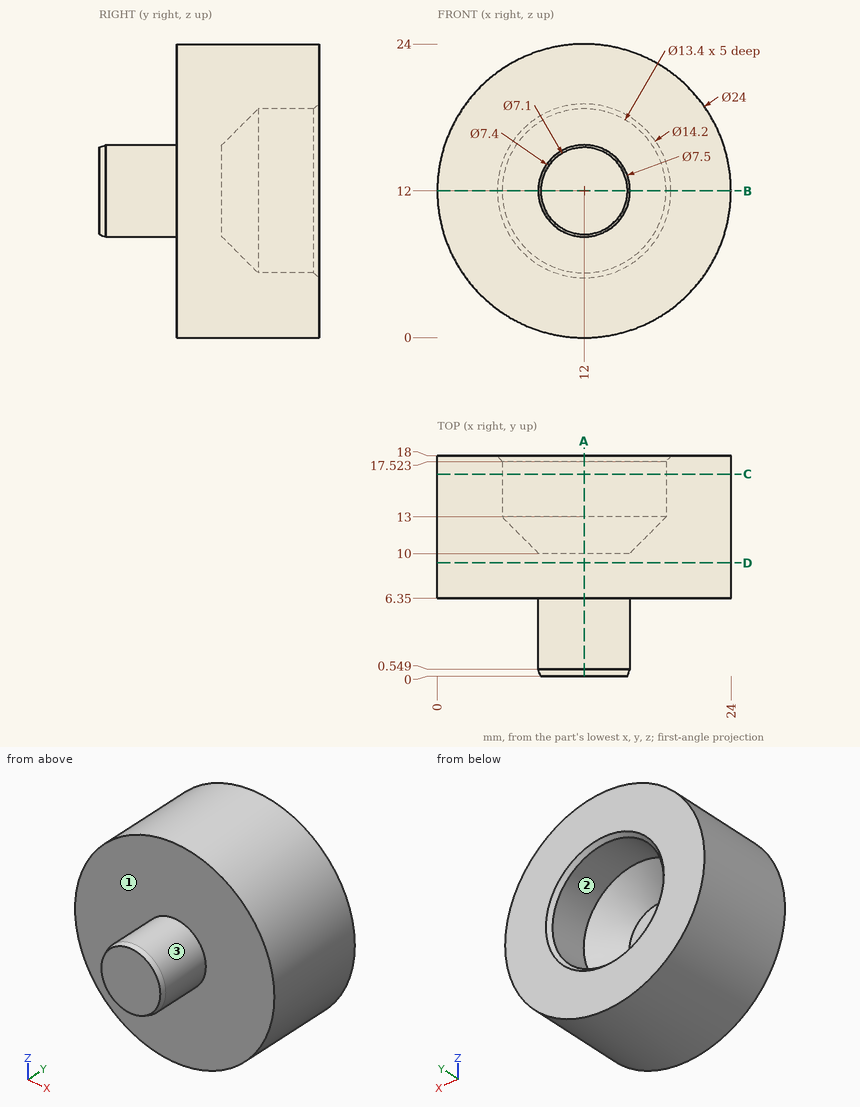
Job drawing, mm, ordinate dimensions from the low corner. One solid piece. Coordinates: 2 decimals unless noted, no trailing zeros. Order: outer loops, then holes, each group sorted by start corner. A loop starts at its lowest first (then second) coordinate and runs counter-clockwise, first axis right, second up. Notation, with made-up numbers: (24.25, 27.25) - (59.25, 27.25) arc R29 ccw to (59.25, 64.25) - close; hole circle Ø1 at (-16, -39.5). An arc over 180 degrees is marked (long way). Use CSV: the item, a comma, the result in double quotes.
Item 1: Drop flat-ended pins along their axis: P1, Ø8, axis at x = 13.5, z = 11, coming from the +Y side; P2, Ø1, axis at x = 7.5, y = 5.5, coming from the -Z side; P3, Ø8, axis at x = 19.5, z = 8, coming from the -Y side; P4, Ø6, axis at y = 15.5, z = 14.5, coming from the -X side. Give the stop position or say it passes through.
Solved:
P1,"stops at y = 12.1"
P2,"passes through"
P3,"stops at y = 6.35"
P4,"stops at x = 0"
Item 2: Saw through at D-D on y = 9.25. Give the cut face in (x, z), and give its area (3 significant figures).
Solved:
outline,"circle Ø24 at (12, 12)"
area,"452 mm²"
Item 3: Saw through at A-A on x = 12. Give the cut face in (y, z), and give its area (3 significant figures).
Solved:
outline,"(0, 8.45) - (0.55, 8.25) - (6.35, 8.25) - (6.35, 0) - (18, 0) - (18, 4.9) - (17.52, 5.3) - (13, 5.3) - (10, 8.3) - (10, 15.7) - (13, 18.7) - (17.52, 18.7) - (18, 19.1) - (18, 24) - (6.35, 24) - (6.35, 15.75) - (0.55, 15.75) - (0, 15.55) - close"
area,"229 mm²"
Item 4: Saw through at B-B on z = 12. Give the cut face in (x, y), and give its area (3 significant figures).
Solved:
outline,"(0, 6.35) - (8.25, 6.35) - (8.25, 0.55) - (8.45, 0) - (15.55, 0) - (15.75, 0.55) - (15.75, 6.35) - (24, 6.35) - (24, 18) - (19.1, 18) - (18.7, 17.52) - (18.7, 13) - (15.7, 10) - (8.3, 10) - (5.3, 13) - (5.3, 17.52) - (4.9, 18) - (0, 18) - close"
area,"229 mm²"
Item 5: Mould opens along Z. For the marked faces 1, 2 and 3 say: +Z half, -Z half, draft (parallel to the pull), parting line (faces both ways), or undercut.
Solved:
face 1,"draft"
face 2,"undercut"
face 3,"parting line"
Item 6: Probe probe 1 along Z at (x, y) = (12, 15.8); probe 2 along Y at (x, z) = (12.5, 10); probe 3 along Z at (x, y) = (8.75, 16.5). List the from-to ranges inside material, lowest first.
Solved:
probe 1,"z = 0 to 5.3, 18.7 to 24"
probe 2,"y = 0 to 10"
probe 3,"z = 0.45 to 6.14, 17.86 to 23.55"
Item 7: Saw through at C-C on y = 16.5. Give the cut face in (x, z).
Solved:
outline,"circle Ø24 at (12, 12); hole circle Ø13.4 at (12, 12)"
